Read the model definition and answer for the solid it produces. Units are mm, in the model's axes. A direction names the side the tool comes from. Coordinates: 2 decimals unless noted, no trailing zeros. Loops run counter-clockwise (first coordinate to the right, second up) from the corner with the lowest first, then second, coordinate; pieces in that order, holes last. Notation, with made-up numbers: (-29, 52.5) - (-23, 52.5) arc R15 ccw to (-23, 66.5) - close; hole circle Ø11 at (64.5, 19.25). An arc over 180 degrees is marked (long way). One line per item, written item: value. Start each with the question number.
from build123d import *

# Parameters (mm, degrees)
F1_DEPTH = 150


with BuildPart() as f1:
    # F0 (on Front) → F1 (new body)
    with BuildSketch(Plane.XZ):
        with BuildLine():
            Line((-43.11781, 78.090709), (-63.11781, 78.090709))
            Line((-63.11781, 78.090709), (-63.11781, 8.090709))
            Line((-63.11781, 8.090709), (286.88219, 8.090709))
            Line((286.88219, 8.090709), (286.88219, 78.090709))
            Line((286.88219, 78.090709), (266.88219, 78.090709))
            ThreePointArc((266.88219, 78.090709), (231.189898, 41.517607), (181.88219, 28.090709))
            Line((181.88219, 28.090709), (111.88219, 28.090709))
            Line((111.88219, 28.090709), (41.88219, 28.090709))
            ThreePointArc((41.88219, 28.090709), (-7.425517, 41.517607), (-43.11781, 78.090709))
        make_face()
    extrude(amount=F1_DEPTH)


solid = f1.part
1) Straight lines are drawn through the part: L1, parallel to Z at x = 180.5, y = -120; L2, parallel to X at y = -17.5, z = 51.5; L3, parallel to X at y = -27, z = 68.5. For each, find the intervals that lie inside material, in ascending order.
2) Section A-A, the plane z = 62 is taken. Determine the outline of the cut face in (x, y).
3) Section D-D, the plane x = 127.5 is taken. Determine the outline of the cut face in (y, z), and give its area (3 significant figures).
4) Section C-C, the plane z = 42.5 is taken. Determine the outline of the cut face in (x, y), and give its area (3 significant figures).
5) Determine the mould class of faces 3 (the flat face through (-63.118, -74, 44)), 4 (the flat face through (113, -74, 28.091)), 5 (the flat face through (277, -74, 78.091)), 6 (the flat face through (286.882, -74, 43)) for opening direction X: released by +X, released by -X, zero draft, split by the parting line, or undercut.
6) Section B-B, the plane y = -62 is taken. Determine the outline of the cut face in (x, z), and give its area (3 significant figures).
7) For faces 1 (the cylindrical face through (232, -74, 42)), 2 (the flat face through (109, -150, 20)), determine the directions among +Z, -Z, +X, -X, +Y, -Y from which every point of the face is accessible in a straight line to the end or side of a thin tool.
8) Flat-ended cylindrical pins translate along their axes: P1, Ø10, axis at x = 217, y = -87, coming from the +Z side; P2, Ø10, axis at x = 39, y = -103.5, coming from the +Z side. Find the tip coordinate at first contact, or state that the pin passes through.
Answer below:
1. L1: 8.09 to 28.09
1. L2: -63.12 to -21.4, 245.17 to 286.88
1. L3: -63.12 to -37.03, 260.79 to 286.88
2. outline: (-63.12, -150) - (-31.91, -150) - (-31.91, 0) - (-63.12, 0) - close; (255.68, -150) - (286.88, -150) - (286.88, 0) - (255.68, 0) - close
3. outline: (-150, 8.09) - (0, 8.09) - (0, 28.09) - (-150, 28.09) - close
3. area: 3,000 mm2
4. outline: (-63.12, -150) - (-9.06, -150) - (-9.06, 0) - (-63.12, 0) - close; (232.82, -150) - (286.88, -150) - (286.88, 0) - (232.82, 0) - close
4. area: 16,200 mm2
5. face 3: released by -X
5. face 4: undercut
5. face 5: zero draft
5. face 6: released by +X
6. outline: (-63.12, 8.09) - (286.88, 8.09) - (286.88, 78.09) - (266.88, 78.09) arc R97.25 cw to (181.88, 28.09) - (41.88, 28.09) arc R97.25 cw to (-43.12, 78.09) - (-63.12, 78.09) - close
6. area: 11,500 mm2
7. face 1: +Z, +Y, -Y
7. face 2: +Z, -Z, +X, -X, -Y
8. P1: z = 36.75
8. P2: z = 28.41
